from build123d import *
from build123d.topology import SkipClean

# Parameters (mm, degrees)
ESBO_O1_W                  = 134
ESBO_O1_H                  = 74
ESBO_O1_W_2                = 130
ESBO_O1_H_2                = 70
RESSALTO_EXTRUS_O1_DEPTH   = 60
ESBO_O2_W                  = 134
ESBO_O2_H                  = 74
ESBO_O2_R                  = 2
RESSALTO_EXTRUS_O2_DEPTH   = 2
ESBO_O3_W                  = 25
ESBO_O3_H                  = 25
ESBO_O3_W_2                = 14
ESBO_O3_H_2                = 16
ESBO_O3_W_3                = 10
ESBO_O3_H_3                = 30
USB_FONTE_DEPTH            = 10
SAIDA_START                = -20
ESBO_O6_W                  = 8
ESBO_O6_H                  = 40
SAIDA_DE_AR_DEPTH          = 97.468879964
ESBO_O7_W                  = 10
ESBO_O7_H                  = 30
DISPLAY_DEPTH              = 12
ESBO_O8_R                  = 4.5
ESBO_O8_R_2                = 1.35
RESSALTO_EXTRUS_O3_DEPTH   = 5
ESBO_O8_3_R                = 1.35
CORTE_EXTRUS_O4_DEPTH      = 97.031244915
CORTE_EXTRUS_O5_DEPTH      = 2
CORTE_EXTRUS_O5_DEPTH_BACK = 10
ESBO_O9_R                  = 3
COOLER_START               = -72
ESBO_O10_R                 = 27.5
ESBO_O10_R_2               = 1
ESBO_O10_W                 = 5
ESBO_O10_H                 = 20
COOLER_DEPTH               = 45.468879964
RESSALTO_EXTRUS_O4_START   = -8
ESBO_O11_R                 = 1.65
RESSALTO_EXTRUS_O4_DEPTH   = 7


with BuildPart() as part:
    # Esboço1 → Ressalto-extrusão1 (new body)
    with BuildSketch(Plane.XY):
        Rectangle(ESBO_O1_W, ESBO_O1_H)
        Rectangle(ESBO_O1_W_2, ESBO_O1_H_2, mode=Mode.SUBTRACT)
    extrude(amount=RESSALTO_EXTRUS_O1_DEPTH)

    # Esboço2 → Ressalto-extrusão2 (add)
    with BuildSketch(Plane(origin=(0, 0, 0), x_dir=(-1, 0, 0), z_dir=(0, 0, -1))):
        Rectangle(ESBO_O2_W, ESBO_O2_H)
        with Locations((-55, -27.5)):
            Circle(ESBO_O2_R, mode=Mode.SUBTRACT)
        with Locations((55, -27.5)):
            Circle(ESBO_O2_R, mode=Mode.SUBTRACT)
        with Locations((55, 27.5)):
            Circle(ESBO_O2_R, mode=Mode.SUBTRACT)
        with Locations((-55, 27.5)):
            Circle(ESBO_O2_R, mode=Mode.SUBTRACT)
    extrude(amount=-RESSALTO_EXTRUS_O2_DEPTH)

    # Esboço3 → USB + fonte (cut)
    with BuildSketch(Plane(origin=(67, 0, 0), x_dir=(0, 0, -1), z_dir=(1, 0, 0))):
        with Locations((-30.5, 10.4)):
            Rectangle(ESBO_O3_W, ESBO_O3_H)
        with Locations((-14, -17.1)):
            Rectangle(ESBO_O3_W_2, ESBO_O3_H_2)
        with Locations((-52, 0)):
            Rectangle(ESBO_O3_W_3, ESBO_O3_H_3)
    extrude(amount=-USB_FONTE_DEPTH, mode=Mode.SUBTRACT)

    # Esboço6 → saida de ar (cut, through all)
    with BuildSketch(Plane.XZ.offset(37).offset(SAIDA_START)):
        with Locations((-48, 30)):
            Rectangle(ESBO_O6_W, ESBO_O6_H)
        with Locations((-35, 30)):
            Rectangle(ESBO_O6_W, ESBO_O6_H)
        with Locations((-22, 30)):
            Rectangle(ESBO_O6_W, ESBO_O6_H)
        with Locations((-9, 30)):
            Rectangle(ESBO_O6_W, ESBO_O6_H)
        with Locations((4, 30)):
            Rectangle(ESBO_O6_W, ESBO_O6_H)
        with Locations((17, 30)):
            Rectangle(ESBO_O6_W, ESBO_O6_H)
        with Locations((30, 30)):
            Rectangle(ESBO_O6_W, ESBO_O6_H)
        with Locations((43, 30)):
            Rectangle(ESBO_O6_W, ESBO_O6_H)
    extrude(amount=-SAIDA_DE_AR_DEPTH, mode=Mode.SUBTRACT)

    # Esboço7 → display (cut)
    with BuildSketch(Plane.ZY.offset(67)):
        with Locations((43, 0)):
            Rectangle(ESBO_O7_W, ESBO_O7_H)
        with Locations((23, 0)):
            Rectangle(ESBO_O7_W, ESBO_O7_H)
    extrude(amount=-DISPLAY_DEPTH, mode=Mode.SUBTRACT)

    # Esboço8 → Ressalto-extrusão3 (add)
    # profile 1 of 3: a face of its own
    with BuildSketch(Plane(origin=(0, 0, 2), x_dir=(-1, 0, 0), z_dir=(0, 0, -1))):
        with Locations(Location((37.3, 20.5, 0), (0, 0, 180))):
            Circle(ESBO_O8_R)
        with Locations(Location((37.3, 20.5, 0), (0, 0, 180))):
            Circle(ESBO_O8_R_2, mode=Mode.SUBTRACT)
    # profile 2 of 3: a face of its own
    with BuildSketch(Plane(origin=(0, 0, 2), x_dir=(-1, 0, 0), z_dir=(0, 0, -1))):
        with Locations(Location((-45, 20.5, 0), (0, 0, 180))):
            Circle(ESBO_O8_R)
        with Locations(Location((-45, 20.5, 0), (0, 0, 180))):
            Circle(ESBO_O8_R_2, mode=Mode.SUBTRACT)
    # profile 3 of 3: a face of its own
    with BuildSketch(Plane(origin=(0, 0, 2), x_dir=(-1, 0, 0), z_dir=(0, 0, -1))):
        with Locations(Location((-43.7, -27.67, 0), (0, 0, 180))):
            Circle(ESBO_O8_R)
        with Locations(Location((-43.7, -27.67, 0), (0, 0, 180))):
            Circle(ESBO_O8_R_2, mode=Mode.SUBTRACT)
    extrude(amount=-RESSALTO_EXTRUS_O3_DEPTH)

    # Esboço8<3> → Corte-extrusão4 (cut, through all)
    with SkipClean():  # the faces are left unmerged after this step: merging them gives an invalid solid
        with BuildSketch(Plane(origin=(0, 0, 2), x_dir=(-1, 0, 0), z_dir=(0, 0, -1))):
            with Locations((-43.7, -27.67)):
                Circle(ESBO_O8_3_R)
            with Locations((37.3, 20.5)):
                Circle(ESBO_O8_3_R)
            with Locations((-45, 20.5)):
                Circle(ESBO_O8_3_R)
        extrude(amount=CORTE_EXTRUS_O4_DEPTH, mode=Mode.SUBTRACT)

    # Esboço9 → Corte-extrusão5 (cut, two sides: drawn at the far end of the back side and taken through both)
    with BuildSketch(Plane.XY.offset(2).offset(-CORTE_EXTRUS_O5_DEPTH_BACK)):
        with Locations((45, 20.5)):
            Circle(ESBO_O9_R)
        with Locations((43.7, -27.67)):
            Circle(ESBO_O9_R)
        with Locations((-37.3, 20.5)):
            Circle(ESBO_O9_R)
    extrude(amount=CORTE_EXTRUS_O5_DEPTH + CORTE_EXTRUS_O5_DEPTH_BACK, mode=Mode.SUBTRACT)

    # Esboço10 → cooler (cut, through all)
    with BuildSketch(Plane(origin=(0, 37, 0), x_dir=(1, 0, 0), z_dir=(0, 1, 0)).offset(COOLER_START)):
        with Locations(Location((32.5, -30, 0), (0, 0, 270))):
            Circle(ESBO_O10_R)
        with Locations(Location((-32.5, -30, 0), (0, 0, 270))):
            Circle(ESBO_O10_R)
        with Locations(Location((-57.5, -55, 0), (0, 0, 270))):
            Circle(ESBO_O10_R_2)
        with Locations(Location((-7.5, -55, 0), (0, 0, 270))):
            Circle(ESBO_O10_R_2)
        with Locations(Location((7.5, -55, 0), (0, 0, 270))):
            Circle(ESBO_O10_R_2)
        with Locations(Location((57.5, -55, 0), (0, 0, 270))):
            Circle(ESBO_O10_R_2)
        with Locations(Location((57.5, -5, 0), (0, 0, 270))):
            Circle(ESBO_O10_R_2)
        with Locations(Location((7.5, -5, 0), (0, 0, 270))):
            Circle(ESBO_O10_R_2)
        with Locations(Location((-7.5, -5, 0), (0, 0, 270))):
            Circle(ESBO_O10_R_2)
        with Locations(Location((-57.5, -5, 0), (0, 0, 270))):
            Circle(ESBO_O10_R_2)
        with Locations((0, -30)):
            Rectangle(ESBO_O10_W, ESBO_O10_H)
    extrude(amount=-COOLER_DEPTH, mode=Mode.SUBTRACT)

    # Esboço11 → Ressalto-extrusão4 (add)
    # profile 1 of 4: a face of its own
    with BuildSketch(Plane.XY.offset(60).offset(RESSALTO_EXTRUS_O4_START)):
        with BuildLine():
            Line((65, -25), (60, -25))
            ThreePointArc((60, -25), (55, -20), (60, -15))
            Line((60, -15), (65, -15))
            Line((65, -15), (65, -25))
        make_face()
        with Locations((60, -20)):
            Circle(ESBO_O11_R, mode=Mode.SUBTRACT)
    # profile 2 of 4: a face of its own
    with BuildSketch(Plane.XY.offset(60).offset(RESSALTO_EXTRUS_O4_START)):
        with BuildLine():
            Line((65, 35), (60, 35))
            ThreePointArc((60, 35), (56.464466094, 26.464466094), (65, 30))
            Line((65, 30), (65, 35))
        make_face()
        with Locations((60, 30)):
            Circle(ESBO_O11_R, mode=Mode.SUBTRACT)
    # profile 3 of 4: a face of its own
    with BuildSketch(Plane.XY.offset(60).offset(RESSALTO_EXTRUS_O4_START)):
        with BuildLine():
            Line((-65, -25), (-65, -15))
            Line((-65, -15), (-60, -15))
            ThreePointArc((-60, -15), (-55, -20), (-60, -25))
            Line((-60, -25), (-65, -25))
        make_face()
        with Locations((-60, -20)):
            Circle(ESBO_O11_R, mode=Mode.SUBTRACT)
    # profile 4 of 4: a face of its own
    with BuildSketch(Plane.XY.offset(60).offset(RESSALTO_EXTRUS_O4_START)):
        with BuildLine():
            Line((-60, 35), (-65, 35))
            Line((-65, 35), (-65, 30))
            ThreePointArc((-65, 30), (-56.464466094, 26.464466094), (-60, 35))
        make_face()
        with Locations((-60, 30)):
            Circle(ESBO_O11_R, mode=Mode.SUBTRACT)
    extrude(amount=-RESSALTO_EXTRUS_O4_DEPTH)


solid = part.part
Here's how the part is built. I have some questions about the finished solid (model axes, mm). A direction names the side the tool comes from. Coordinates: 2 decimals unless noted, no trailing zeros. Loops run counter-clockwise (first coordinate to the right, second up) from the corner with the lowest first, then second, coordinate; pieces in that order, holes last.
1. Imagine slicing it at C-C, the plane y = -20. Please give me the cut outline in (x, z), and give its area (3 significant figures).
2. Imagine slicing it at A-A, the plane y = 4. Please give me the cut outline in (x, z).
3. I need wall thicknesses on L1, parallel to X at y = 34.5, z = 41.5; L2, parallel to Y at x = -54.5, z = 49.5; L3, parallel to X at y = -17.5, z = 9. Which ranges of each line are inside material? Lowest first, please.
4. Imagine slicing it at B-B, the plane x = -49.5. Please give me the cut outline in (y, z), and give its area (3 significant figures).
5. For P1, Ø1, axis at x = 38, y = 16.5, coming from the +Z side; P2, Ø7, axis at x = -39, y = 20, coming from the +Z side; P3, Ø4, axis at x = -34.5, z = 40.5, coming from the -Y side, each with a flat end and sliding along its axis, tell me the tip position at first contact or that it passes through.
6. If we mould it in two halves opening along X, with no side actions, what happens to faces 5 (the flat face through (-1, -37, 16)), 6 (the cylindrical face through (55.434, -29.452, 0.986))? For each: pulls with the +X half, pulls with the -X half, needs draft (parallel to the pull), parting line crosses it, or undercut.
7. Imagine slicing it at D-D, the plane x = -15.5. Please give me the cut outline in (y, z).
8. For faces 1 (the flat face through (-62, -25, 49)), 2 (the flat face through (-62, -20, 45)), 3 (the cylindrical face through (-54.566, -29.452, 0.986)), 4 (the cylindrical face through (42, 20.6, 2)), which set-ups out of +Z, -Z, +X, -X, +Y, -Y let a thin tool reach every point of the face, with its end or its side?
Taken from the geometry:
1. outline: (-67, 0) - (67, 0) - (67, 7) - (65, 7) - (65, 2) - (-65, 2) - (-65, 45) - (-61.65, 45) - (-61.65, 52) - (-65, 52) - (-65, 60) - (-67, 60) - close; (-58.35, 45) - (-55, 45) - (-55, 52) - (-58.35, 52) - close; (55, 45) - (58.35, 45) - (58.35, 52) - (55, 52) - close; (61.65, 45) - (65, 45) - (65, 21) - (67, 21) - (67, 60) - (65, 60) - (65, 52) - (61.65, 52) - close
1. area: 566 mm2
2. outline: (-67, 0) - (67, 0) - (67, 18) - (65, 18) - (65, 2) - (-65, 2) - (-65, 18) - (-67, 18) - close; (-67, 28) - (-65, 28) - (-65, 38) - (-67, 38) - close; (-67, 48) - (-65, 48) - (-65, 60) - (-67, 60) - close; (65, 43) - (67, 43) - (67, 47) - (65, 47) - close; (65, 57) - (67, 57) - (67, 60) - (65, 60) - close
3. L1: x = -67 to -65, 65 to 67
3. L2: y = -37 to -35, 35 to 37
3. L3: x = -67 to -65
4. outline: (-37, 0) - (37, 0) - (37, 10) - (35, 10) - (35, 2) - (-35, 2) - (-35, 8.38) - (-37, 8.38) - close; (-37, 51.62) - (-35, 51.62) - (-35, 60) - (-37, 60) - close; (35, 50) - (37, 50) - (37, 60) - (35, 60) - close
4. area: 214 mm2
5. P1: stops at z = 2
5. P2: stops at z = 7
5. P3: passes through
6. face 5: needs draft
6. face 6: undercut
7. outline: (-37, 0) - (37, 0) - (37, 60) - (35, 60) - (35, 2) - (-35, 2) - (-35, 8.38) - (-37, 8.38) - close; (-37, 51.62) - (-35, 51.62) - (-35, 60) - (-37, 60) - close
8. face 1: +Z
8. face 2: none
8. face 3: +Z, -Z
8. face 4: -Z
